```python
from build123d import *

# Parameters (mm, degrees)
SKETCH4_R                = 1.65
CUT_EXTRUDE4_DEPTH       = 21.784609691
SKETCH5_OUTSIDE_W        = 33.422
SKETCH5_OUTSIDE_H        = 33.422
CUT_EXTRUDE5_DEPTH       = 21.784609691
CUT_EXTRUDE2_DEPTH       = 16
BOSS_EXTRUDE1_REACH      = 27.258
BOSS_EXTRUDE1_END_RADIUS = 5
SKETCH3_R                = 2.75
CUT_EXTRUDE6_REACH       = 27.258
SKETCH6_R                = 1.6
FILLET1_R                = 1
CHAMFER1_SIZE            = 0.5
FILLET2_R                = 1


with BuildPart() as part:
    # Sketch1 → Revolve1 (revolve)
    with BuildSketch(Plane(origin=(0, 0, 0), x_dir=(0, 0, -1), z_dir=(1, 0, 0))):
        Polygon((0, 0), (12, 0), (12, 3), (5, 3), (5, 15), (0, 15), (0, 5.353547723), align=None)
    revolve(axis=Axis((0, 5.353547723, 0), (0, 1, 0)))

    # Sketch4 → Cut-Extrude4 (cut, through all)
    with BuildSketch(Plane(origin=(0, 3, 0), x_dir=(1, 0, 0), z_dir=(0, 1, 0))):
        with Locations(Location((0, 8.5, 0), (0, 0, 270))):
            Circle(SKETCH4_R)
        with Locations(Location((7.361215932, -4.25, 0), (0, 0, 270))):
            Circle(SKETCH4_R)
        with Locations(Location((-7.361215932, -4.25, 0), (0, 0, 270))):
            Circle(SKETCH4_R)
    extrude(amount=-CUT_EXTRUDE4_DEPTH, mode=Mode.SUBTRACT)

    # Sketch5 outside → Cut-Extrude5 (cut, through all)
    with BuildSketch(Plane(origin=(0, 3, 0), x_dir=(1, 0, 0), z_dir=(0, 1, 0))):
        Rectangle(SKETCH5_OUTSIDE_W, SKETCH5_OUTSIDE_H)
        with BuildLine():
            Line((-3.031088913, 10.25), (-10.392304845, -2.5))
            ThreePointArc((-10.392304845, -2.5), (-10.392304845, -6), (-7.361215932, -7.75))
            Line((-7.361215932, -7.75), (7.361215932, -7.75))
            ThreePointArc((7.361215932, -7.75), (10.392304845, -6), (10.392304845, -2.5))
            Line((10.392304845, -2.5), (3.031088913, 10.25))
            ThreePointArc((3.031088913, 10.25), (0, 12), (-3.031088913, 10.25))
        make_face(mode=Mode.SUBTRACT)
    extrude(amount=-CUT_EXTRUDE5_DEPTH, mode=Mode.SUBTRACT)

    # Sketch2 → Cut-Extrude2 (cut)
    with BuildSketch(Plane(origin=(0, 15, 0), x_dir=(1, 0, 0), z_dir=(0, 1, 0))):
        Polygon((2.886751346, 0), (1.443375673, 2.5), (-1.443375673, 2.5), (-2.886751346, 0), (-1.443375673, -2.5), (1.443375673, -2.5), align=None)
    extrude(amount=-CUT_EXTRUDE2_DEPTH, mode=Mode.SUBTRACT)

    # Boss-Extrude1: up to this cylinder (the profile starts outside it)
    boss_extrude1_end = Plane(origin=(0, 9, 0), z_dir=(0, -1, 0)) * Cylinder(BOSS_EXTRUDE1_END_RADIUS, 65.516, mode=Mode.PRIVATE)
    # Sketch3 → Boss-Extrude1 (add, up to the surface)
    with BuildSketch(Plane(origin=(6.062177826, 0, -3.5), x_dir=(-0.5000000000000001, 0, -0.8660254037844386), z_dir=(0.8660254037844386, 0, -0.5000000000000001)), mode=Mode.PRIVATE) as boss_extrude1_sk1:
        with Locations((0, 9)):
            Circle(SKETCH3_R)
    boss_extrude1_tool1 = extrude(boss_extrude1_sk1.sketch, amount=-BOSS_EXTRUDE1_REACH, mode=Mode.PRIVATE) - boss_extrude1_end
    add(boss_extrude1_tool1.solids().sort_by_distance((6.062178, 9, -3.5))[0])

    # Sketch6 → Cut-Extrude6 (cut, up to next)
    with BuildSketch(Plane(origin=(6.062177826, 0, -3.5), x_dir=(-0.5000000000000001, 0, -0.8660254037844386), z_dir=(0.8660254037844386, 0, -0.5000000000000001)), mode=Mode.PRIVATE) as cut_extrude6_sk1:
        with Locations((0, 9)):
            Circle(SKETCH6_R)
    cut_extrude6_tool1 = extrude(cut_extrude6_sk1.sketch, amount=-CUT_EXTRUDE6_REACH, mode=Mode.PRIVATE) & part.part
    add(cut_extrude6_tool1.solids().sort_by_distance((6.062178, 9, -3.5))[0], mode=Mode.SUBTRACT)

    # Fillet1
    fillet1_edges = [part.edges().sort_by_distance(p)[0] for p in [
        (0, 3, 5),
    ]]
    fillet(fillet1_edges, radius=FILLET1_R)

    # Chamfer1
    chamfer1_edges = [part.edges().sort_by_distance(p)[0] for p in [
        (6.862177826, 9, -2.114359354),
    ]]
    chamfer(chamfer1_edges, length=CHAMFER1_SIZE)

    # Fillet2
    fillet2_edges = [part.edges().sort_by_distance(p)[0] for p in [
        (4.991369035, 8.999999998, 0.293658225),
    ]]
    fillet(fillet2_edges, radius=FILLET2_R)


solid = part.part
```
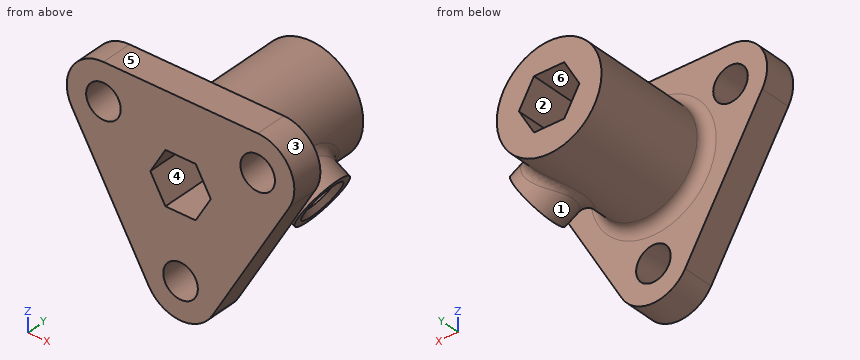
Part model, mm, in its own coordinate system. Face numbers are marked on the shaded views. A direction names the side the tool comes from. Give positions to 0.01 mm unless a question says otherwise; leave off trailing zeros. Write each loop counter-clockwise with the first axis right and the second up, starting at its lowest first coordinate (ties: lowest second). Pieces come first, ordered by that corner, then holes. Notation, with made-up numbers: (44.5, 20) -> (62.5, 20) arc R28 cw to (62.5, 53) -> close; hole circle Ø2 at (78.25, 25.5). An arc over 180 degrees is marked (long way). Put each result on its own line as item: value. Start each with the question number.
Item 1: Which spindle directions (+Z, -Z, +X, -X, +Y, -Y) get a long thin tool onto all of the face, cutting with end or side? Do the marked faces 1 and 2. Say none if no direction does.
Item 2: Pin check, flat tips, straight feed: pin 1 Ø1 at (x, y) = (1, 9) entering from -Z; pin 2 Ø10 at (x, z) = (6.5, 3.5) entering from +Y; pin 3 Ø5.5 at (x, z) = (0, -8.5) entering from +Y; pin 4 Ø2.5 at (x, y) = (-0.5, 7) entering from +Z. Stop position of each tip, or through.
Item 3: Cut at D-D (z = -8.5). List the corners of the cut face in (x, y), then the cut area to 3 significant figures.
Item 4: Pull direction X, two halves, no side cores. Call the marked faces 3, 4, 5 and 6: pulls with the +X half, pulls with the -X half, needs draft (parallel to the pull), parting line crosses it, or undercut.
Item 5: Wall check: L1, parallel to X at y = 1.7, z = 4.25; L2, parallel to Z at x = 8.25, y = 0.5; L3, parallel to Y at x = 2.25, z = 7. Give the ranges that are in metal, low to high. Write a range as [from, to].
Item 6: Cut at C-C (y = 13.25). List the corners of the cut face in (x, z).
Item 7: Cut at B-B (y = 1). List the corners of the cut face in (x, z), then the cut area to 3 significant figures.
Item 8: Cut at A-A (x = 0). List the corners of the cut face in (y, z).
Answer list:
1. face 1: none
1. face 2: +Y, -Y
2. pin 1: stops at z = -4.97
2. pin 2: stops at y = 15
2. pin 3: stops at y = 3.03
2. pin 4: stops at z = 5
3. outline: (-4.04, 0) -> (-1.65, 0) -> (-1.65, 3) -> (-4.04, 3) -> close; (1.65, 0) -> (4.04, 0) -> (4.04, 3) -> (1.65, 3) -> close
3. area: 14.3 mm2
4. face 3: pulls with the +X half
4. face 4: undercut
4. face 5: needs draft
4. face 6: undercut
5. L1: x = [-10.86, -9.01], [-5.71, 5.71], [9.01, 10.86]
5. L2: z = [-1.21, 2.86], [5.64, 7.64]
5. L3: y = [0, 3]
6. outline: circle Ø10 at (0, 0); hole (-2.89, 0) -> (-1.44, -2.5) -> (1.44, -2.5) -> (2.89, 0) -> (1.44, 2.5) -> (-1.44, 2.5) -> close
7. outline: (-10.39, 2.5) -> (-3.03, -10.25) arc R3.5 ccw to (3.03, -10.25) -> (10.39, 2.5) arc R3.5 ccw to (7.36, 7.75) -> (-7.36, 7.75) arc R3.5 ccw to start; hole circle Ø3.3 at (-7.36, 4.25); hole (-2.89, 0) -> (-1.44, -2.5) -> (1.44, -2.5) -> (2.89, 0) -> (1.44, 2.5) -> (-1.44, 2.5) -> close; hole circle Ø3.3 at (0, -8.5); hole circle Ø3.3 at (7.36, 4.25)
7. area: 240 mm2
8. outline: (0, -12) -> (3, -12) -> (3, -10.15) -> (0, -10.15) -> close; (0, -6.85) -> (3, -6.85) -> (3, -6) arc R1 cw to (4, -5) -> (15, -5) -> (15, -2.5) -> (0, -2.5) -> close; (0, 2.5) -> (15, 2.5) -> (15, 5) -> (4, 5) arc R1 cw to (3, 6) -> (3, 7.75) -> (0, 7.75) -> close
